Can you work these out from the model? Positions are in its coordinate system, mm. A direction names the side the tool comes from. Round coordinates to 2 decimals unless told otherwise and drop trailing zeros. Loops run counter-clockwise (first coordinate to the right, second up) from the corner with the lowest first, then second, coordinate; pieces in that order, holes last. Notation, with made-up numbers: (58, 23) - (98, 23) arc R11 ccw to (98, 31) - close; hole circle Ø5 at (75.5, -24). An arc over 180 degrees is marked (long way). Answer as CSV lines item,"result".
```python
from build123d import *

# Parameters (mm, degrees)
SKETCH3_R           = 2.5
BOSS_EXTRUDE1_DEPTH = 3
FILLET1_R           = 5


with BuildPart() as part:
    # Sketch1 → Revolve1 (revolve)
    with BuildSketch(Plane.XY, mode=Mode.PRIVATE) as revolve1_sk:
        with BuildLine():
            Line((0, 4.25), (0, -25.75))
            Line((0, -25.75), (-2.5, -25.75))
            Line((-2.5, -25.75), (-2.5, -3.436931771))
            ThreePointArc((-2.5, -3.436931771), (-4.041624675, 1.314446646), (0, 4.25))
        make_face()
    revolve(revolve1_sk.sketch.rotate(Axis((0, 4.25, 0), (0, -1, 0)), 180), axis=Axis((0, 4.25, 0), (0, -1, 0)))

    # Sketch3 → Boss-Extrude1 (add)
    with BuildSketch(Plane(origin=(0, -25.75, 0), x_dir=(-1, 0, 0), z_dir=(0, -1, 0))):
        with BuildLine():
            Line((8.378284652, 45), (8.378284652, 0))
            ThreePointArc((8.378284652, 0), (0, -8.378284652), (-8.378284652, 0))
            Line((-8.378284652, 0), (-8.378284652, 45))
            ThreePointArc((-8.378284652, 45), (0, 53.378284652), (8.378284652, 45))
        make_face()
        with Locations(Location((0, 45, 0), (0, 0, 180))):
            Circle(SKETCH3_R, mode=Mode.SUBTRACT)
    extrude(amount=BOSS_EXTRUDE1_DEPTH)

    # Fillet1
    fillet1_edges = [part.edges().sort_by_distance(p)[0] for p in [
        (-2.5, -25.75, 0),
        (-2.5, -3.436931771, 0),
    ]]
    fillet(fillet1_edges, radius=FILLET1_R)


solid = part.part
```
Q1. We'd pull the mould along X, two halves only. Please class faces 1 (the flat face through (8.378, -27, -22)), 2 (the cylindrical face through (-0.54, -27.23, -47.44)), 3 (the flat face through (-8.378, -27, -23)), 4 (the flat face through (0, -25.75, -30)): pulls with the +X half, pulls with the -X half, needs draft (parallel to the pull), parting line crosses it, or undercut.
Checks:
face 1,"pulls with the +X half"
face 2,"undercut"
face 3,"pulls with the -X half"
face 4,"needs draft"
Q2. On a 3-axis mill with a long thin cutter (end or side, diameter ignored), from which of +Z, -Z, +X, -X, +Y, -Y can I reach the whole of each face in a straight line? I mean faces 5 (the cylindrical face through (0.184, -27.229, -53.376)), 6 (the cylindrical face through (-2.5, -13, 0.1)). Say none if no direction works.
Checks:
face 5,"-Z, +Y, -Y"
face 6,"none"
Q3. If I drill on line 1 along Z through (x, y) = (0, -26.45); line 2 along Y through (x, z) = (-0.5, -29.5); line 3 along Z through (x, y) = (-1.5, -6.5), over which ranges is the centre line in solid material (lowest first)? Write a range as [from, to].
Checks:
line 1,"[-53.38, -47.5], [-42.5, 8.38]"
line 2,"[-28.75, -25.75]"
line 3,"[-2, 2]"
Q4. I'm going to push flat-ended pins straight in: pin 1 Ø8.5 at (x, z) = (3, -27.5) entering from +Y; pin 2 Ø5 at (x, y) = (-6, -19) entering from +Z; pin 3 Ø8 at (y, z) = (-13, -3) entering from +X. Where does each tip first touch, or does it pass through?
Checks:
pin 1,"y = -25.75"
pin 2,"through"
pin 3,"x = 2.5"
Q5. Imagine slicing it at B-B (z = -12). Write out the boundary of the cut face in (x, y), then the cut area to 3 significant figures.
Checks:
outline,"(-8.38, -28.75) - (8.38, -28.75) - (8.38, -25.75) - (-8.38, -25.75) - close"
area,"50.3 mm²"
Q6. Imagine slicing it at A-A (y = -14). Write out the boundary of the cut face in (x, z), then the cut area to 3 significant figures.
Checks:
outline,"circle Ø5 at (0, 0)"
area,"19.6 mm²"
